The listing builds one solid part. Answer for the finished solid, in the listing's coordinates (mm). A direction names the side the tool comes from. Give positions to 0.01 mm unless a question says otherwise; leave off trailing zeros. Order: outer loops, then holes, each group sorted by start corner. A loop starts at its lowest first (then second) coordinate and runs counter-clockwise, first axis right, second up. Notation, with made-up numbers: (26.5, 69.25) -> (51.5, 69.25) arc R25 cw to (51.5, 99.25) -> close; hole circle Ø1 at (-21, 72). An arc over 180 degrees is marked (long way). Answer as a JSON object with one key per item and string values. Group by question number.
```python
from build123d import *

# Parameters (mm, degrees)
BOSS_EXTRUDE1_DEPTH      = 10
SKETCH2_R                = 40
BOSS_EXTRUDE2_DEPTH      = 10
SKETCH3_R                = 30
CUT_EXTRUDE1_DEPTH       = 10
SKETCH4_R                = 10
CUT_EXTRUDE2_DEPTH       = 10
BOSS_EXTRUDE4_DEPTH      = 5
BOSS_EXTRUDE4_DEPTH_BACK = 55
SKETCH5_R                = 10


with BuildPart() as part:
    # Sketch1 → Boss-Extrude1 (new body)
    with BuildSketch(Plane(origin=(0, 0, 0), x_dir=(1, 0, 0), z_dir=(0, 1, 0))):
        with BuildLine():
            Line((-200, 40), (0, 40))
            ThreePointArc((0, 40), (40, 0), (0, -40))
            Line((0, -40), (-200, -40))
            ThreePointArc((-200, -40), (-240, 0), (-200, 40))
        make_face()
    extrude(amount=BOSS_EXTRUDE1_DEPTH)

    # Sketch2 → Boss-Extrude2 (add)
    with BuildSketch(Plane(origin=(0, 10, 0), x_dir=(1, 0, 0), z_dir=(0, 1, 0))):
        with Locations(Location((-200, 0, 0), (0, 0, 270))):
            Circle(SKETCH2_R)
    extrude(amount=BOSS_EXTRUDE2_DEPTH)

    # Sketch3 → Cut-Extrude1 (cut)
    with BuildSketch(Plane(origin=(0, 20, 0), x_dir=(1, 0, 0), z_dir=(0, 1, 0))):
        with Locations(Location((-200, 0, 0), (0, 0, 270))):
            Circle(SKETCH3_R)
    extrude(amount=-CUT_EXTRUDE1_DEPTH, mode=Mode.SUBTRACT)

    # Sketch4 → Cut-Extrude2 (cut)
    with BuildSketch(Plane(origin=(0, 10, 0), x_dir=(1, 0, 0), z_dir=(0, 1, 0))):
        with Locations(Location((-200, 0, 0), (0, 0, 270))):
            Circle(SKETCH4_R)
    extrude(amount=-CUT_EXTRUDE2_DEPTH, mode=Mode.SUBTRACT)

    # Sketch5 → Boss-Extrude4 (add, two sides: drawn at the far end of the back side and taken through both)
    with BuildSketch(Plane(origin=(0, 10, 0), x_dir=(1, 0, 0), z_dir=(0, 1, 0)).offset(-BOSS_EXTRUDE4_DEPTH_BACK)):
        with Locations(Location((0, 0, 0), (0, 0, 270))):
            Circle(SKETCH5_R)
    extrude(amount=BOSS_EXTRUDE4_DEPTH + BOSS_EXTRUDE4_DEPTH_BACK)


solid = part.part
```
(1) A cutting plane is placed at C-C (y = -29.5). Determine the outline of the cut face in (x, z).
(2) Flat-ended cylindrical pins translate along their axes: pin 1 Ø23 at (x, z) = (-200, 0) entering from +Y; pin 2 Ø2 at (y, z) = (0.5, 14.5) entering from +X; pin 3 Ø1.5 at (x, z) = (-117.5, 18) entering from -Y. Find the tip coordinate at first contact, or state that the pin passes through.
(3) A cutting plane is placed at B-B (x = -205.5). Determine the outline of the cut face in (y, z).
(4) Find the intervals of material crossed by line 1 along X through (y, z) = (12.75, 0); line 2 along X through (y, z) = (7, 0); line 3 along Y through (x, z) = (-189.5, -35), in increasing order. Write a range as [from, to].
(5) A cutting plane is placed at A-A (z = 0). Determine the outline of the cut face in (x, y), and give its area (3 significant figures).
(6) For a pull along Z with two mould halves and no side action, classify faces 1 (the cylindrical face through (39.99, 4.93, -0.88)), 2 (the cylindrical face through (-209.76, 5.07, -2.17)), 3 (the flat face through (-78, 10, -1)) as +Z half, -Z half, draft (parallel to the pull), parting line (faces both ways), or undercut.
(7) A cutting plane is placed at D-D (x = 7). Determine the outline of the cut face in (y, z).
(8) Which of the six approach directions +Z, -Z, +X, -X, +Y, -Y give full straight-line access (tool end or side, diameter ignored) to faces 4 (the flat face through (-99, 5, 40)), 5 (the cylindrical face through (-9.76, -22.82, -2.17)), 6 (the flat face through (-101, 5, -40)), 7 (the flat face through (0, 15, 0)), 8 (the cylindrical face through (-229.287, 15.07, -6.503))?
Check sheet entries:
{
 "1": {"outline": "circle Ø20 at (0, 0)"},
 "2": {"pin 1": "stops at y = 10", "pin 2": "stops at x = 37.65", "pin 3": "stops at y = 0"},
 "3": {"outline": "(0, -39.62) -> (20, -39.62) -> (20, -29.49) -> (10, -29.49) -> (10, -8.35) -> (0, -8.35) -> close; (0, 8.35) -> (10, 8.35) -> (10, 29.49) -> (20, 29.49) -> (20, 39.62) -> (0, 39.62) -> close"},
 "4": {"line 1": "x = [-240, -230], [-170, -160], [-10, 10]", "line 2": "x = [-240, -210], [-190, 40]", "line 3": "y = [0, 20]"},
 "5": {"outline": "(-240, 0) -> (-210, 0) -> (-210, 10) -> (-230, 10) -> (-230, 20) -> (-240, 20) -> close; (-190, 0) -> (-10, 0) -> (-10, -45) -> (10, -45) -> (10, 0) -> (40, 0) -> (40, 10) -> (10, 10) -> (10, 15) -> (-10, 15) -> (-10, 10) -> (-160, 10) -> (-160, 20) -> (-170, 20) -> (-170, 10) -> (-190, 10) -> close", "area": "3,800 mm2"},
 "6": {"face 1": "parting line", "face 2": "undercut", "face 3": "draft"},
 "7": {"outline": "(-45, -7.14) -> (0, -7.14) -> (0, -39.38) -> (10, -39.38) -> (10, -7.14) -> (15, -7.14) -> (15, 7.14) -> (10, 7.14) -> (10, 39.38) -> (0, 39.38) -> (0, 7.14) -> (-45, 7.14) -> close"},
 "8": {"face 4": "+Z, +X, -X, +Y, -Y", "face 5": "-Y", "face 6": "-Z, +X, -X, +Y, -Y", "face 7": "+Z, -Z, +X, +Y", "face 8": "+Y"}
}
